Geometry: final body of the model. Coordinates: model frame, mm. Round coordinates to 2 decimals unless told otherwise and drop trailing zeros. Order: outer loops, then holes, each group sorted by start corner. A loop starts at its lowest first (then second) coordinate and runs counter-clockwise, first axis right, second up. Notation, with made-up numbers: (21.25, 31.5) - (46.25, 31.5) arc R36 cw to (46.25, 68.5) - close; hole circle Ø9 at (-30, 68.25). An arc over 180 degrees is marked (long way). Put each result on its own line as item: value. Start each with the question number.
(1) Material intervals for L1, parallel to X at y = 5, z = 0; L2, parallel to X at y = 12, z = 0; L3, parallel to Y at x = 10, z = -1.5, sorted ascending. Write a range as [from, to].
(2) Section D-D (x = 60). Output: boundary loops of the cut face in (y, z), and give its area (3 significant figures).
(3) Pin query (flat end, axial travel): P1, Ø12, axis at y = 1.5, z = 1.5, coming from the +X side; P2, Ø1.5, axis at x = 52.5, y = 6, coming from the -Z side; P3, Ø11, axis at x = 4.5, z = -7.5, coming from the -Y side; P4, Ø4, axis at x = 47, z = 12, coming from the +Y side. Return the tip coordinate at first contact, or that it passes through.
(4) Section B-B (x = 0). Output: boundary loops of the cut face in (y, z).
(5) Section C-C (z = 4). Output: boundary loops of the cut face in (x, y).
(6) Section A-A (z = 0). Output: boundary loops of the cut face in (x, y).
(7) Pull-direction query (X, two-part tool) for faces 1 (the face through (-4, 24, 8)), 2 (the face through (-17.572, 14.499, -3.902)), 3 (the face through (31.28, 4.93, -14.45)), 4 (the face through (55.043, -2.675, 0.651)); classes: released by +X, released by -X, zero draft, split by the parting line, or undercut.
from build123d import *

# Parameters (mm, degrees)
SKETCH_1_R          = 18
EXTRUDE_1_DEPTH     = 24
EXTRUDE_2_DEPTH     = 10
EXTRUDE_START       = -15
SKETCH_3_R          = 11
EXTRUDE_3_DEPTH     = 15
SKETCH_4_R          = 8
CUT_EXTRUDE_1_DEPTH = 83.981925743
SKETCH_5_R          = 5
CUT_EXTRUDE_2_DEPTH = 83.981925743


with BuildPart() as part:
    # 草图1 → 凸台-拉伸1 (new body)
    with BuildSketch(Plane(origin=(0, 0, 0), x_dir=(1, 0, 0), z_dir=(0, 1, 0))):
        with Locations(Location((0, 0, 0), (0, 0, 270))):
            Circle(SKETCH_1_R)
    extrude(amount=EXTRUDE_1_DEPTH)

    # 草图2 → 凸台-拉伸2 (add)
    with BuildSketch(Plane(origin=(0, 0, 0), x_dir=(1, 0, 0), z_dir=(0, 1, 0))):
        with BuildLine():
            Line((2.1, 17.877080299), (61.283333333, 10.924882405))
            ThreePointArc((61.283333333, 10.924882405), (71, 0), (61.283333333, -10.924882405))
            Line((61.283333333, -10.924882405), (2.1, -17.877080299))
            ThreePointArc((2.1, -17.877080299), (-18, 0), (2.1, 17.877080299))
        make_face()
    extrude(amount=EXTRUDE_2_DEPTH)

    # 草图3 → 凸台-拉伸3 (add)
    with BuildSketch(Plane(origin=(0, 0, 0), x_dir=(1, 0, 0), z_dir=(0, 1, 0)).offset(EXTRUDE_START)):
        with Locations(Location((60, 0, 0), (0, 0, 83.300234822))):
            Circle(SKETCH_3_R)
    extrude(amount=EXTRUDE_3_DEPTH)

    # 草图4 → 切除-拉伸1 (cut, through all)
    with BuildSketch(Plane(origin=(0, 24, 0), x_dir=(1, 0, 0), z_dir=(0, 1, 0))):
        with Locations(Location((0, 0, 0), (0, 0, 270))):
            Circle(SKETCH_4_R)
    extrude(amount=-CUT_EXTRUDE_1_DEPTH, mode=Mode.SUBTRACT)

    # 草图5 → 切除-拉伸2 (cut, through all)
    with BuildSketch(Plane(origin=(0, -15, 0), x_dir=(1, 0, 0), z_dir=(0, 1, 0))):
        with Locations(Location((60, 0, 0), (0, 0, 90))):
            Circle(SKETCH_5_R)
    extrude(amount=CUT_EXTRUDE_2_DEPTH, mode=Mode.SUBTRACT)


solid = part.part
Checks:
1. L1: x = [-18, -8], [8, 55], [65, 71]
1. L2: x = [-18, -8], [8, 18]
1. L3: y = [0, 24]
2. outline: (-15, -11) - (0, -11) - (0, -11.08) - (10, -11.08) - (10, -5) - (-15, -5) - close; (-15, 5) - (10, 5) - (10, 11.08) - (0, 11.08) - (0, 11) - (-15, 11) - close
2. area: 302 mm²
3. P1: stops at x = 71
3. P2: stops at z = -12.04
3. P3: stops at y = 0
3. P4: stops at y = 10
4. outline: (0, -18) - (24, -18) - (24, -8) - (0, -8) - close; (0, 8) - (24, 8) - (24, 18) - (0, 18) - close
5. outline: (-17.55, 0) - (-6.93, 0) - (-6.93, 24) - (-17.55, 24) - close; (6.93, 0) - (49.75, 0) - (49.75, -15) - (57, -15) - (57, 10) - (17.55, 10) - (17.55, 24) - (6.93, 24) - close; (63, -15) - (70.25, -15) - (70.25, 10) - (63, 10) - close
6. outline: (-18, 0) - (-8, 0) - (-8, 24) - (-18, 24) - close; (8, 0) - (49, 0) - (49, -15) - (55, -15) - (55, 10) - (18, 10) - (18, 24) - (8, 24) - close; (65, -15) - (71, -15) - (71, 10) - (65, 10) - close
7. face 1: zero draft
7. face 2: split by the parting line
7. face 3: released by +X
7. face 4: undercut
